Source: CAD feature listing. Evaluate the final solid. Frame: model axes, mm. A direction names the side the tool comes from. Coordinates: 2 decimals unless noted, no trailing zeros. Loops run counter-clockwise (first coordinate to the right, second up) from the corner with the lowest first, then second, coordinate; pieces in that order, holes last.
Item 1: Pull-direction query (X, two-part tool) for faces 1 (the flat face through (111, 221, -2898.727)), 2 (the conical face through (-29.509, 326.025, -2505.033)), 3 (the cylindrical face through (36.354, 370.293, -2579.966)), 4 (the conical face through (-87.319, 140.974, -2787.679)); classes: +X half, -X half, draft (parallel to the pull), parting line (faces both ways), or undercut.
Item 2: Section query B-B, the plane z = -2630.5. Return the cut outline in (x, y).
Item 3: Section query C-C, the plane y = 286.5. State how many separate pieces and enclosed holes the cut face has, then the cut area to 3 significant figures.
Item 4: Reachability of faces 5 (the flat face through (-56, 195, -2433.826)), 6 (the cylindrical face through (-50.18, 375.89, -2574.45)), 7 (the flat face through (-67, 357, -2888.727)) from +Z, -Z, +X, -X, +Y, -Y: full face, straight path, thin tool, end or side. Return the list, or none.
Item 5: Section query D-D, the plane z = -2754. Return the cut outline in (x, y).
Item 6: Line query: probe 1 along X at (y, z) = (256.5, -2661); probe 2 along X at (y, z) = (309, -2513); probe 3 along Y at (x, z) = (-27.5, -2794). Output: solid intervals per line, ascending.
Item 7: Section query A-A, the plane x = 0. Return the cut outline in (y, z).
Item 8: Pin query (flat end, axial travel): pin 1 Ø1.5 at (y, z) = (179, -2772.5) entering from -X; pin 2 Ø6 at (y, z) = (203, -2672.5) entering from -X; pin 3 Ø6 at (x, z) = (-7.5, -2497) entering from -Y. Return the tip coordinate at first contact, or that it passes through.
```python
from build123d import *


with BuildPart() as part:
    # Sketch1 → Revolve-Thin1 (revolve)
    with BuildSketch(Plane(origin=(0, 0, 0), x_dir=(0, 0, -1), z_dir=(1, 0, 0))):
        Polygon((2433.826246914, 385.88150306), (2433.826246914, 334.771392049), (2541.94019818, 314.975879845), (2735.520516837, 314.975879845), (2898.727447068, 368.64302357), (2898.727447068, 418.546471621), (2719.070119986, 385.88150306), align=None)
        Polygon((2443.826246914, 375.88150306), (2443.826246914, 343.106649757), (2542.848144127, 324.975879845), (2733.918565509, 324.975879845), (2888.727447068, 375.88150306), (2888.727447068, 406.56434445), (2719.971819423, 375.88150306), align=None, mode=Mode.SUBTRACT)
    revolve(axis=Axis((0, 254.852892636, -1616.565391775), (0, 0, -1)))


solid = part.part
```
Verdict:
1. face 1: draft
1. face 2: undercut
1. face 3: undercut
1. face 4: parting line
2. outline: circle Ø262.06 at (0, 254.85); circle Ø140.25 at (0, 254.85); hole circle Ø242.06 at (0, 254.85); hole circle Ø120.25 at (0, 254.85)
3. separate pieces: 2
3. enclosed holes: 2
3. area: 21,500 mm2
4. face 5: +Z, +X, -X, +Y, -Y
4. face 6: +Z
4. face 7: none
5. outline: circle Ø274.76 at (0, 254.85); circle Ø153.45 at (0, 254.85); hole circle Ø254.43 at (0, 254.85); hole circle Ø132.4 at (0, 254.85)
6. probe 1: x = -131.02 to -121.02, -70.1 to -60.1, 60.1 to 70.1, 121.02 to 131.02
6. probe 2: x = -119.32 to -108.24, -52.74 to -36.72, 36.72 to 52.74, 108.24 to 119.32
6. probe 3: y = 112.84 to 123.21, 169.28 to 180.42, 329.29 to 340.42, 386.5 to 396.87
7. outline: (91.16, -2898.73) - (141.06, -2898.73) - (194.73, -2735.52) - (194.73, -2541.94) - (174.93, -2433.83) - (123.82, -2433.83) - (123.82, -2719.07) - close; (314.98, -2735.52) - (368.64, -2898.73) - (418.55, -2898.73) - (385.88, -2719.07) - (385.88, -2433.83) - (334.77, -2433.83) - (314.98, -2541.94) - close; hole (103.14, -2888.73) - (133.82, -2888.73) - (184.73, -2733.92) - (184.73, -2542.85) - (166.6, -2443.83) - (133.82, -2443.83) - (133.82, -2719.97) - close; hole (324.98, -2733.92) - (375.88, -2888.73) - (406.56, -2888.73) - (375.88, -2719.97) - (375.88, -2443.83) - (343.11, -2443.83) - (324.98, -2542.85) - close
8. pin 1: stops at x = -119.06
8. pin 2: stops at x = -121.58
8. pin 3: stops at y = 123.9
